from build123d import *

# Parameters (mm, degrees)
ESQUISSE1_W        = 50
ESQUISSE1_H        = 50
ESQUISSE1_W_2      = 36
ESQUISSE1_H_2      = 6
ESQUISSE1_W_3      = 10
ESQUISSE1_H_3      = 8
ESQUISSE1_W_4      = 45
BOSS_EXTRU_1_DEPTH = 5
ESQUISSE11_W       = 10
ESQUISSE11_H       = 5
BOSS_EXTRU_2_DEPTH = 5


with BuildPart() as part:
    # Esquisse1 → Boss.-Extru.1 (new body)
    with BuildSketch(Plane.XY):
        with Locations((-25, 25)):
            Rectangle(ESQUISSE1_W, ESQUISSE1_H)
        with Locations((-25, 41)):
            Rectangle(ESQUISSE1_W_2, ESQUISSE1_H_2, mode=Mode.SUBTRACT)
        with Locations((-25, 21.5)):
            Rectangle(ESQUISSE1_W_3, ESQUISSE1_H_3, mode=Mode.SUBTRACT)
        with Locations((-25, 10)):
            Rectangle(ESQUISSE1_W_4, ESQUISSE1_H_3, mode=Mode.SUBTRACT)
    extrude(amount=BOSS_EXTRU_1_DEPTH)

    # Esquisse11 → Boss.-Extru.2 (add)
    with BuildSketch(Plane.XY.offset(5)):
        with Locations((-35, -2.5)):
            Rectangle(ESQUISSE11_W, ESQUISSE11_H)
        with Locations((-15, -2.5)):
            Rectangle(ESQUISSE11_W, ESQUISSE11_H)
    extrude(amount=-BOSS_EXTRU_2_DEPTH)


solid = part.part
Design review of the part built by this model. Coordinates are the model's own, in mm. A direction names the side the tool comes from. Give positions to 0.01 mm unless a question says otherwise; leave off trailing zeros. Order: outer loops, then holes, each group sorted by start corner. A loop starts at its lowest first (then second) coordinate and runs counter-clockwise, first axis right, second up. Notation, with made-up numbers: (43.25, 54) - (88.25, 54) arc R32 cw to (88.25, 89) - close; hole circle Ø11 at (-36.75, 70). An arc over 180 degrees is marked (long way). Use CSV: the item, a comma, the result in double quotes. Start each with the question number.
Q1. Take a section at C-C (x = -16). State the section outline as (y, z) points, and give its area (3 significant figures).
Q2. Take a section at D-D (z = 0.8). State the section outline as (x, y) points, and give its area (3 significant figures).
Q3. For P1, Ø2.5, axis at x = -25.5, z = 2.5, coming from the -Y side, flat-tipped, find the tip position at first contact; note if it passes through.
Q4. Take a section at B-B (y = 19). State the section outline as (x, z) points.
Q5. Machinability: for faces 4 (the face through (-5, 0, 2)), 5 (the face through (-30, -3, 3)), 6 (the face through (-25, 44, 2)), which of the approach directions +Z, -Z, +X, -X, +Y, -Y give a long, thin tool a straight path to every point of the face, cutting with its end or side? Answer none if there is none.
Q6. For line 1 (Y direction, x = -8.5, z = 3.95); line 2 (Y direction, x = -27.5, z = 2.05); line 3 (Y direction, x = -3, z = 3.85), list the stretches that pass through material, from the lowest coordinate up.
Q7. Take a section at A-A (x = -22). State the section outline as (y, z) points, and give its area (3 significant figures).
Q8. Draft analysis for pull direction Y (two halves, no side actions). For faces 1 (the face through (-25, 6, 2)), 2 (the face through (-25, 50, 2)), 3 (the face through (0, 25, 2)), state which applies: pulls with the +Y half, pulls with the -Y half, needs draft (parallel to the pull), parting line crosses it, or undercut.
Calculated:
1,outline,"(-5, 0) - (6, 0) - (6, 5) - (-5, 5) - close; (14, 0) - (38, 0) - (38, 5) - (14, 5) - close; (44, 0) - (50, 0) - (50, 5) - (44, 5) - close"
1,area,"205 mm²"
2,outline,"(-50, 0) - (-40, 0) - (-40, -5) - (-30, -5) - (-30, 0) - (-20, 0) - (-20, -5) - (-10, -5) - (-10, 0) - (0, 0) - (0, 50) - (-50, 50) - close; hole (-47.5, 6) - (-2.5, 6) - (-2.5, 14) - (-47.5, 14) - close; hole (-43, 38) - (-7, 38) - (-7, 44) - (-43, 44) - close; hole (-30, 17.5) - (-20, 17.5) - (-20, 25.5) - (-30, 25.5) - close"
2,area,"1,940 mm²"
3,P1,"stops at y = 0"
4,outline,"(-50, 0) - (-30, 0) - (-30, 5) - (-50, 5) - close; (-20, 0) - (0, 0) - (0, 5) - (-20, 5) - close"
5,face 4,"+Z, -Z, +X, -Y"
5,face 5,"+Z, -Z, -Y"
5,face 6,"+Z, -Z"
6,line 1,"y = 0 to 6, 14 to 38, 44 to 50"
6,line 2,"y = 0 to 6, 14 to 17.5, 25.5 to 38, 44 to 50"
6,line 3,"y = 0 to 6, 14 to 50"
7,outline,"(0, 0) - (6, 0) - (6, 5) - (0, 5) - close; (14, 0) - (17.5, 0) - (17.5, 5) - (14, 5) - close; (25.5, 0) - (38, 0) - (38, 5) - (25.5, 5) - close; (44, 0) - (50, 0) - (50, 5) - (44, 5) - close"
7,area,"140 mm²"
8,face 1,"undercut"
8,face 2,"pulls with the +Y half"
8,face 3,"needs draft"
